from build123d import *


with BuildPart() as part:
    # Çizim1 → Döndür1 (revolve)
    with BuildSketch(Plane.XY, mode=Mode.PRIVATE) as d_nd_r1_sk:
        Polygon((-150, 40), (0, 40), (0, 36), (-20, 36), (-20, 35), (-130, 35), (-130, 36), (-150, 36), align=None)
    revolve(d_nd_r1_sk.sketch.rotate(Axis((-88.99, 0, 0), (1, 0, 0)), 90), axis=Axis((-88.99, 0, 0), (1, 0, 0)))


solid = part.part
Input: part model. Units: mm. Frame: model coordinates. A direction names the side the tool comes from. Round coordinates to 2 decimals unless told otherwise and drop trailing zeros. Order: outer loops, then holes, each group sorted by start corner. A loop starts at its lowest first (then second) coordinate and runs counter-clockwise, first axis right, second up. Notation, with made-up numbers: (35.5, 67.25) - (81.5, 67.25) arc R22 cw to (81.5, 99.25) - close; hole circle Ø1 at (59, 79.25). An arc over 180 degrees is marked (long way). Use a Markdown table: item, result.
1. Section C-C on x = -64. Return the cut outline in (y, z).
Evaluation:
| item | result |
|---|---|
| outline | circle Ø80 at (0, 0); hole circle Ø70 at (0, 0) |
2. Section A-A on y = 0. Return the cut outline in (x, z).
Evaluation:
| item | result |
|---|---|
| outline | (-150, -40) - (0, -40) - (0, -36) - (-20, -36) - (-20, -35) - (-130, -35) - (-130, -36) - (-150, -36) - close; (-150, 36) - (-130, 36) - (-130, 35) - (-20, 35) - (-20, 36) - (0, 36) - (0, 40) - (-150, 40) - close |
3. First-contact query: pin 1 (2 mm diameter, centred on x = -33, z = 18.5, fed in from -Y); pin 2 (3 mm diameter, centred on x = -113.5, y = 29.5, fed in from +Z); pin 3 (3 mm diameter, centred on x = -87.5, y = 12, fed in from -Z). Flat tips, straight axial feed; report the tip coordinate or a pass-through.
Evaluation:
| item | result |
|---|---|
| pin 1 | y = -35.97 |
| pin 2 | z = 28.57 |
| pin 3 | z = -38.6 |
4. Access query for faces 5 (the face through (-20, -19, -30)), 6 (the face through (-130, -19, 30)), 7 (the face through (-150, -15, 33)). Directions: +Z, -Z, +X, -X, +Y, -Y. A direction counts if a zero-diameter tool reaches every point of the face in a straight line with its end or side. Return the directions, or none.
Evaluation:
| item | result |
|---|---|
| face 5 | +X |
| face 6 | -X |
| face 7 | +Z, -Z, -X, +Y, -Y |
5. Mould query, pull axis Z, two halves, no side actions, for faces 1 (the face through (-75.77, 34.168, -7.587)), 2 (the face through (0, -15, -33)), 3 (the face through (-140.14, -24.331, -26.533)), 4 (the face through (-73.95, -1.76, -39.96)). Classes: +Z half, -Z half, draft (parallel to the pull), parting line (faces both ways), or undercut.
Evaluation:
| item | result |
|---|---|
| face 1 | undercut |
| face 2 | draft |
| face 3 | undercut |
| face 4 | parting line |
6. Material intervals for probe 1 along Y at (x, z) = (-90.5, 0); probe 2 along Y at (x, z) = (-14, 0); probe 3 along Z at (x, y) = (-19.5, 19), sorted ascending.
Evaluation:
| item | result |
|---|---|
| probe 1 | -40 to -35, 35 to 40 |
| probe 2 | -40 to -36, 36 to 40 |
| probe 3 | -35.2 to -30.58, 30.58 to 35.2 |
